Geometry: final body of the model. Coordinates: model frame, mm. A direction names the side the tool comes from. Give positions to 0.01 mm unless a question says otherwise; leave off trailing zeros. Order: outer loops, then holes, each group sorted by start corner. A loop starts at its lowest first (then second) coordinate and runs counter-clockwise, first axis right, second up. Notation, with made-up numbers: (-30.75, 62.25) - (26.25, 62.25) arc R21 cw to (26.25, 75.25) - close; hole circle Ø1 at (84.25, -38.5). An arc over 180 degrees is marked (long way). One line per item, written item: value.
```python
from build123d import *

# Parameters (mm, degrees)
F1_DEPTH = 25.4
F2_DEPTH = 25.4
F4_DEPTH = 68.58


with BuildPart() as f1:
    # F0 (on Top) → F1 (new body)
    with BuildSketch(Plane.XY):
        Polygon((16.782857, 38.1), (0, 38.1), (0, 12.7), (16.782857, 12.7), (16.782857, 0), (29.482857, 0), (29.482857, 50.8), (16.782857, 50.8), align=None)
        Polygon((54.882857, 50.8), (29.482857, 50.8), (29.482857, 0), (54.882857, 0), (54.882857, 12.7), (50.20391, 12.7), (50.20391, 38.099997), (54.882857, 38.099997), align=None)
    extrude(amount=F1_DEPTH)

    # F1_face (on face) → F2 (join)
    with BuildSketch(Plane(origin=(29.731958, 25.4, 25.4), x_dir=(1, 0, 0), z_dir=(0, 0, 1))):
        Polygon((-12.949101, 25.4), (-12.949101, 12.7), (-29.731958, 12.7), (-29.731958, -12.7), (-12.949101, -12.7), (-12.949101, -25.4), (25.150899, -25.4), (25.150899, -12.7), (20.471952, -12.7), (20.471952, 12.699997), (25.150899, 12.699997), (25.150899, 25.4), align=None)
    extrude(amount=F2_DEPTH)

    # F3 (on face) → F4 (cut)
    with BuildSketch(Plane.XZ):
        Polygon((54.882857, 50.8), (26.128728, 50.8), (54.882857, 18.009631), align=None)
    extrude(amount=-F4_DEPTH, mode=Mode.SUBTRACT)


solid = f1.part
```
1) Material intervals for line 1 along Y through (x, z) = (13, 37); line 2 along X through (y, z) = (17.5, 7.5); line 3 along X through (y, z) = (5, 2), sorted ascending.
Answers below:
line 1: 12.7 to 38.1
line 2: 0 to 50.2
line 3: 16.78 to 54.88
2) Section A-A, the plane y = 8. Return loops of the section in (x, z).
Answers below:
outline: (16.78, 0) - (54.88, 0) - (54.88, 18.01) - (26.13, 50.8) - (16.78, 50.8) - close
3) Mould query, pull axis Y, two halves, no side actions, for faces 6 (the face through (53, 12.7, 12)), 7 (the face through (8, 12.7, 25)), 8 (the face through (40.305, 25.044, 34.634)). Classes: released by +Y, released by -Y, zero draft, split by the parting line, or undercut.
Answers below:
face 6: undercut
face 7: released by -Y
face 8: zero draft
4) Section C-C, the plane x = 4.5. Return loops of the section in (y, z), then the cut area to 3 significant figures.
Answers below:
outline: (12.7, 0) - (38.1, 0) - (38.1, 50.8) - (12.7, 50.8) - close
area: 1,290 mm^2
5) Section D-D, the plane z = 45.5. Return loops of the section in (x, y).
Answers below:
outline: (0, 12.7) - (16.78, 12.7) - (16.78, 0) - (30.78, 0) - (30.78, 50.8) - (16.78, 50.8) - (16.78, 38.1) - (0, 38.1) - close
6) Section B-B, the plane z = 17. Return loops of the section in (x, y).
Answers below:
outline: (0, 12.7) - (16.78, 12.7) - (16.78, 0) - (54.88, 0) - (54.88, 12.7) - (50.2, 12.7) - (50.2, 38.1) - (54.88, 38.1) - (54.88, 50.8) - (16.78, 50.8) - (16.78, 38.1) - (0, 38.1) - close
7) Set-up query: faces 1 (the face through (50.204, 25, 12)), 2 (the face through (16.783, 45, 25)), 3 (the face through (16.783, 6, 25)), 4 (the face through (32, 50.8, 19)), 5 (the face through (54.883, 6, 9)). Return all of +Z, -Z, +X, -X, +Y, -Y with unobstructed straight access to the full face (end or side cutting, diameter ignored); none if empty.
Answers below:
face 1: +Z, -Z, +X
face 2: +Z, -Z, -X, +Y
face 3: +Z, -Z, -X, -Y
face 4: +Z, -Z, +X, -X, +Y
face 5: +Z, -Z, +X, +Y, -Y
8) First-contact query: pin 1 (18.5 mm diameter, centred on x = 7.5, z = 31.5, fed in from -Y); pin 2 (3 mm diameter, centred on x = 33, y = 10, fed in from +Z); pin 3 (5 mm diameter, centred on x = 8, z = 15, fed in from +Y). Flat tips, straight axial feed; report the tip coordinate or a pass-through.
Answers below:
pin 1: y = 12.7
pin 2: z = 44.67
pin 3: y = 38.1
